The listing builds one solid part. Answer for the finished solid, in the listing's coordinates (mm). A direction names the side the tool comes from. Give positions to 0.01 mm unless a question says otherwise; leave off trailing zeros. Order: outer loops, then holes, each group sorted by start corner. A loop starts at its lowest first (then second) coordinate and runs counter-clockwise, first axis right, second up. Notation, with made-up numbers: (-2, 15) - (52, 15) arc R25 cw to (52, 42) - close; hole circle Ø10 at (69.5, -27.75). An arc over 180 degrees is marked (long way). Answer in a Markdown table with one row per item. Add a question column.
```python
from build123d import *

# Parameters (mm, degrees)
PAD_DEPTH       = 10
PAD001_DEPTH    = 80
SKETCH003_R     = 8
POCKET_DEPTH    = 5
SKETCH004_R     = 6
POCKET001_DEPTH = 5
FILLET_R        = 1


with BuildPart() as part:
    # Sketch → Pad (new body)
    with BuildSketch(Plane.XY):
        with BuildLine():
            Line((40, 0), (-40, 0))
            Line((-40, 0), (-40, 15))
            Line((-9.661357, 48.698171), (-40, 15))
            ThreePointArc((9.661357, 48.698171), (0, 53), (-9.661357, 48.698171))
            Line((9.661357, 48.698171), (40, 15))
            Line((40, 0), (40, 15))
        make_face()
    extrude(amount=PAD_DEPTH)

    # Sketch002 (on Face7 of Pad) → Pad001 (join)
    with BuildSketch(Plane(origin=(0, 0, 0), x_dir=(1, 0, 0), z_dir=(0, 0, -1))):
        Polygon((-40, -15), (-40, 0), (-25, 0), (-25, -10), (-30, -10), (-30, -5), (-35, -5), (-35, -15), align=None)
        Polygon((40, -15), (40, 0), (25, 0), (25, -10), (30, -10), (30, -5), (35, -5), (35, -15), align=None)
    extrude(amount=PAD001_DEPTH)

    # Sketch003 (on Face9 of Pad001) → Pocket (cut)
    with BuildSketch(Plane.YZ.offset(40)):
        with Locations((0, -35)):
            Circle(SKETCH003_R)
    extrude(amount=-POCKET_DEPTH, mode=Mode.SUBTRACT)

    # Sketch004 (on Face28 of Pocket) → Pocket001 (cut)
    with BuildSketch(Plane.YZ.offset(-25)):
        with Locations((0, -35)):
            Circle(SKETCH004_R)
    extrude(amount=-POCKET001_DEPTH, mode=Mode.SUBTRACT)

    # Fillet
    fillet_edges = [part.edges().sort_by_distance(p)[0] for p in [
        (37.5, 0, -27),
        (0, 0, 0),
    ]]
    fillet(fillet_edges, radius=FILLET_R)


solid = part.part
```
(1) Straight lines are drawn through the part: line 1 (X direction, y = 6.5, z = -39.5); line 2 (X direction, y = 12.5, z = -54); line 3 (Y direction, x = -34.5, z = -25.5). For each, find the intervals that lie inside material, in ascending order.
(2) Each of these flat-tipped pins is pushed along its axis until it touches: P1, Ø5, axis at x = 22, y = 29.5, coming from the -Z side; P2, Ø1.5, axis at x = -37, z = -52, coming from the +Y side; P3, Ø4, axis at x = 32.5, z = -53, coming from the +Y side; P4, Ø11, axis at y = 5, z = -36.5, coming from the +X side. Where does it stop, or does it pass through?
(3) The mould has two halves that part along Z. Classify faces 1 (the face through (34, 4, -80)), 2 (the face through (37.535, 7.976, -35.614)), 3 (the face through (-24.618, 32.085, 4.93)), 4 (the face through (-27, 6, -35)): +Z half, -Z half, draft (parallel to the pull), parting line (faces both ways), or undercut.
(4) Find section D-D, the plane y = 35.5. Write down the section's boundary in (x, z), plus the area to 3 significant figures.
(5) For faces 5 (the face through (35, 2, -34)), 6 (the face through (37, 15, -39)), 7 (the face through (-32, 5, -39)), determine the directions among +Z, -Z, +X, -X, +Y, -Y from which every point of the face is accessible in a straight line to the end or side of a thin tool.
(6) Find section B-B, the plane z = -24. Write down the section's boundary in (x, y).
(7) Find section A-A, the plane z = -35. Write down the section's boundary in (x, y).
(8) Find section C-C, the plane x = -12. Write down the section's boundary in (y, z).
Answer key:
| question | item | result |
|---|---|---|
| 1 | line 1 | -40 to -35, -30 to -25, 25 to 30 |
| 1 | line 2 | -40 to -35, 35 to 40 |
| 1 | line 3 | 0 to 5 |
| 2 | P1 | z = 0 |
| 2 | P2 | y = 15 |
| 2 | P3 | y = 5 |
| 2 | P4 | x = 40 |
| 3 | face 1 | -Z half |
| 3 | face 2 | undercut |
| 3 | face 3 | draft |
| 3 | face 4 | undercut |
| 4 | outline | (-21.54, 0) - (21.54, 0) - (21.54, 10) - (-21.54, 10) - close |
| 4 | area | 431 mm² |
| 5 | face 5 | +X, -Y |
| 5 | face 6 | -Z, +X, -X, +Y |
| 5 | face 7 | -Z, +Y |
| 6 | outline | (-40, 0) - (-25, 0) - (-25, 10) - (-30, 10) - (-30, 5) - (-35, 5) - (-35, 15) - (-40, 15) - close; (25, 0) - (40, 0) - (40, 15) - (35, 15) - (35, 5) - (30, 5) - (30, 10) - (25, 10) - close |
| 7 | outline | (-40, 0) - (-30, 0) - (-30, 5) - (-35, 5) - (-35, 15) - (-40, 15) - close; (-30, 6) - (-25, 6) - (-25, 10) - (-30, 10) - close; (25, 0) - (35, 0) - (35, 5) - (30, 5) - (30, 10) - (25, 10) - close; (35, 8) - (40, 8) - (40, 15) - (35, 15) - close |
| 8 | outline | (0, 1) arc R1 ccw to (1, 0) - (46.1, 0) - (46.1, 10) - (0, 10) - close |
